```python
from build123d import *

# Parameters (mm, degrees)
SKETCH1_R             = 12.75
BOSS_EXTRUDE1_DEPTH   = 5
SKETCH2_R             = 6
BOSS_EXTRUDE2_DEPTH   = 4.25
SKETCH3_R             = 3
CUT_EXTRUDE1_DEPTH    = 10.25
F_4_40_TAPPED_HOLE2_D = 2.2606


with BuildPart() as part:
    # Sketch1 → Boss-Extrude1 (new body)
    with BuildSketch(Plane(origin=(0, 0, 0), x_dir=(1, 0, 0), z_dir=(0, 1, 0))):
        Circle(SKETCH1_R)
    extrude(amount=BOSS_EXTRUDE1_DEPTH)

    # Sketch2 → Boss-Extrude2 (add)
    with BuildSketch(Plane(origin=(0, 5, 0), x_dir=(1, 0, 0), z_dir=(0, 1, 0))):
        Circle(SKETCH2_R)
    extrude(amount=BOSS_EXTRUDE2_DEPTH)

    # Sketch3 → Cut-Extrude1 (cut, through all)
    with BuildSketch(Plane(origin=(0, 9.25, 0), x_dir=(1, 0, 0), z_dir=(0, 1, 0))):
        Circle(SKETCH3_R)
    extrude(amount=-CUT_EXTRUDE1_DEPTH, mode=Mode.SUBTRACT)

    # #4-40 Tapped Hole2 (through all)
    with Locations(Plane(origin=(0, 5, 0), x_dir=(1, 0, 0), z_dir=(0, 1, 0))):
        with Locations((-4.609677481, -8.277058611), (-9.525, 0), (4.7625, -8.248891971), (9.525, 0), (-4.7625, 8.248891971), (4.7625, 8.248891971)):
            Hole(F_4_40_TAPPED_HOLE2_D / 2)


solid = part.part
```
Source: CAD feature listing. Evaluate the final solid. Frame: model axes, mm. A direction names the side the tool comes from. Coordinates: 2 decimals unless noted, no trailing zeros. Loops run counter-clockwise (first coordinate to the right, second up) from the corner with the lowest first, then second, coordinate; pieces in that order, holes last. Notation, with made-up numbers: M 69,87.25 L 76,87.25 A20 ccw 76,116.25 Z; hole C 58,48 d6. An arc over 180 degrees is marked long. Use CSV: the item, a comma, the result in double quotes.
(1) Line query: line 1 (Z direction, x = 0, y = 4); line 2 (X direction, y = 7, z = 0); line 3 (Y direction, x = 8.25, z = 2.25). Output: solid intervals per line, ascending. Write a range as [from, to].
Answers follow:
line 1,"[-12.75, -3], [3, 12.75]"
line 2,"[-6, -3], [3, 6]"
line 3,"[0, 5]"
(2) Cut plane C-C on y = 3.5. Give the number of separate pieces and of enclosed holes in the cut face, and give its area (3 significant figures).
Answers follow:
separate pieces,"1"
enclosed holes,"7"
area,"458 mm²"
(3) Reachability of faces 1 (the face through (-3, 5, 5.5)), 2 (the face through (10.654, 2.465, -0.05)) from +Z, -Z, +X, -X, +Y, -Y: full face, straight path, thin tool, end or side. Return the list, or none.
Answers follow:
face 1,"+Y"
face 2,"+Y, -Y"
(4) Draft query along X for faces 3 (the face through (-3, 9.25, 1)), 4 (the face through (5.01, 2.46, 9.35)), 5 (the face through (-2.764, 2.465, 12.447)). Return one class per face: pulls with the +X half, pulls with the -X half, needs draft (parallel to the pull), parting line crosses it, or undercut.
Answers follow:
face 3,"needs draft"
face 4,"undercut"
face 5,"parting line crosses it"
(5) Contact query for flat-ended pins moving along their axis: pin 1 (1.8 mm diameter, centred on x = 9.525, z = 0, fed in from +Y); pin 2 (3 mm diameter, centred on x = -4.76, z = -8.25, fed in from +Y); pin 3 (1 mm diameter, centred on x = 4.5, y = 7.5, fed in from -Z). Output: stop coordinate, or through.
Answers follow:
pin 1,"through"
pin 2,"y = 5"
pin 3,"z = -4.47"
(6) Cut plane D-D on z = -3.5. Return loops of the section in (x, y), and give its area (3 significant figures).
Answers follow:
outline,"M -12.26,0 L 12.26,0 L 12.26,5 L 4.87,5 L 4.87,9.25 L -4.87,9.25 L -4.87,5 L -12.26,5 Z"
area,"164 mm²"
(7) Cut plane A-A on x = 0. Return loops of the section in (y, z), and give its area (3 significant figures).
Answers follow:
outline,"M 0,-12.75 L 5,-12.75 L 5,-6 L 9.25,-6 L 9.25,-3 L 0,-3 Z; M 0,3 L 9.25,3 L 9.25,6 L 5,6 L 5,12.75 L 0,12.75 Z"
area,"123 mm²"
(8) Cut plane B-B on z = 0. Return loops of the section in (x, y).
Answers follow:
outline,"M -12.75,0 L -10.66,0 L -10.66,5 L -12.75,5 Z; M -8.39,0 L -3,0 L -3,9.25 L -6,9.25 L -6,5 L -8.39,5 Z; M 3,0 L 8.39,0 L 8.39,5 L 6,5 L 6,9.25 L 3,9.25 Z; M 10.66,0 L 12.75,0 L 12.75,5 L 10.66,5 Z"
